The listing builds one solid part. Answer for the finished solid, in the listing's coordinates (mm). A direction names the side the tool comes from. Round coordinates to 2 decimals unless told otherwise and drop trailing zeros. Write each loop counter-clockwise with the first axis right and the second up, starting at its lowest first coordinate (ties: lowest second). Pieces come first, ordered by that corner, then holes. Notation, with made-up numbers: (10.5, 8.25) - (30.5, 8.25) arc R18 cw to (30.5, 12.25) - close; hole circle Ø7 at (-39.5, 83). An arc over 180 degrees is marked (long way). Use a Markdown table: item, result. Add a question column.
1) A cutting plane is placed at A-A (z = 2.25). Give the vertices of the cut face in (x, y), then the cut area to 3 significant figures.
2) A tool of negligible diameter and unlimited length cuts with its end or side. For faces 1 (the cylindrical face through (-0.54, -2.44, 3.48)), 2 (the flat face through (-6, 0, 1)), from which of +Z, -Z, +X, -X, +Y, -Y can it reach the whole face along a straight path? Write none if from no direction.
3) Find the intervals of material crossed by probe 1 along Y at (x, z) = (0, 4.15); probe 2 along Z at (x, y) = (-1, 3.5); probe 3 along X at (y, z) = (-1, 3.8), in increasing order. Write a range as from..to.
4) Determine the mould class of faces 3 (the cylindrical face through (-3, 0, 3)), 4 (the flat face through (0, 0, 2)), 5 (the flat face through (0, 6, 1)) for opening direction X: +X half, -X half, draft (parallel to the pull), parting line (faces both ways), or undercut.
5) A cutting plane is placed at D-D (y = 2.75). Give the vertices of the cut face in (x, z), then the cut area to 3 significant figures.
6) Each of these flat-tipped pins is pushed along its axis until it touches: P1, Ø2, axis at y = -2.5, z = 3.5, coming from the +X side; P2, Ø1, axis at y = -3, z = 3.5, coming from the -X side. Where does it stop, or does it pass through?
7) A cutting plane is placed at B-B (x = 0). Give the vertices of the cut face in (y, z), then the cut area to 3 significant figures.
```python
from build123d import *

# Parameters (mm, degrees)
SKETCH1_W           = 12
SKETCH1_H           = 12
BOSS_EXTRUDE1_DEPTH = 2
SKETCH2_R           = 3
SKETCH2_R_2         = 2.5
BOSS_EXTRUDE2_DEPTH = 3


with BuildPart() as part:
    # Sketch1 → Boss-Extrude1 (new body)
    with BuildSketch(Plane.XY):
        Rectangle(SKETCH1_W, SKETCH1_H)
    extrude(amount=BOSS_EXTRUDE1_DEPTH)

    # Sketch2 → Boss-Extrude2 (add)
    with BuildSketch(Plane.XY.offset(2)):
        Circle(SKETCH2_R)
        Circle(SKETCH2_R_2, mode=Mode.SUBTRACT)
    extrude(amount=BOSS_EXTRUDE2_DEPTH)


solid = part.part
```
Entries:
| question | item | result |
|---|---|---|
| 1 | outline | circle Ø6 at (0, 0); hole circle Ø5 at (0, 0) |
| 1 | area | 8.64 mm² |
| 2 | face 1 | +Z |
| 2 | face 2 | +Z, -Z, -X, +Y, -Y |
| 3 | probe 1 | y = -3..-2.5, 2.5..3 |
| 3 | probe 2 | z = 0..2 |
| 3 | probe 3 | x = -2.83..-2.29, 2.29..2.83 |
| 4 | face 3 | parting line |
| 4 | face 4 | undercut |
| 4 | face 5 | draft |
| 5 | outline | (-6, 0) - (6, 0) - (6, 2) - (1.2, 2) - (1.2, 5) - (-1.2, 5) - (-1.2, 2) - (-6, 2) - close |
| 5 | area | 31.2 mm² |
| 6 | P1 | stops at x = 2.6 |
| 6 | P2 | stops at x = -1.66 |
| 7 | outline | (-6, 0) - (6, 0) - (6, 2) - (3, 2) - (3, 5) - (2.5, 5) - (2.5, 2) - (-2.5, 2) - (-2.5, 5) - (-3, 5) - (-3, 2) - (-6, 2) - close |
| 7 | area | 27.0 mm² |
